The listing builds one solid part. Answer for the finished solid, in the listing's coordinates (mm). Face numbers are marked on the shaded views. Give positions to 0.01 mm unless a question says otherwise; leave off trailing zeros. Loops run counter-clockwise (first coordinate to the right, second up) from the corner with the lowest first, then second, coordinate; pieces in that order, holes last. Notation, with made-up numbers: (30, 6) -> (44, 6) arc R22 cw to (44, 40) -> close; hole circle Ø6 at (-32, 85.25). An arc over 180 degrees is marked (long way). One line per question, with ' | ' between items. Start each with the question number.
from build123d import *

# Parameters (mm, degrees)
SKETCH_1_W          = 206
SKETCH_1_H          = 215
EXTRUDE_1_DEPTH     = 15
SHELL_1_T           = -2
SKETCH_2_R          = 3
CUT_EXTRUDE_1_DEPTH = 15


with BuildPart() as part:
    # 草图1 → 凸台-拉伸1 (new body)
    with BuildSketch(Plane.XY):
        Rectangle(SKETCH_1_W, SKETCH_1_H)
    extrude(amount=EXTRUDE_1_DEPTH)

    # 抽壳1
    shell_1_openings = [part.faces().sort_by_distance(p)[0] for p in [
        (0, 0, 15),
    ]]
    offset(amount=SHELL_1_T, openings=shell_1_openings, kind=Kind.INTERSECTION)

    # 草图2 → 切除-拉伸1 (cut)
    with BuildSketch(Plane.XY.offset(2)):
        with Locations((-92, 0)):
            Circle(SKETCH_2_R)
        with Locations((0, 96.5)):
            Circle(SKETCH_2_R)
        with Locations((92, 0)):
            Circle(SKETCH_2_R)
        with Locations((0, -96.5)):
            Circle(SKETCH_2_R)
    extrude(amount=-CUT_EXTRUDE_1_DEPTH, mode=Mode.SUBTRACT)


solid = part.part
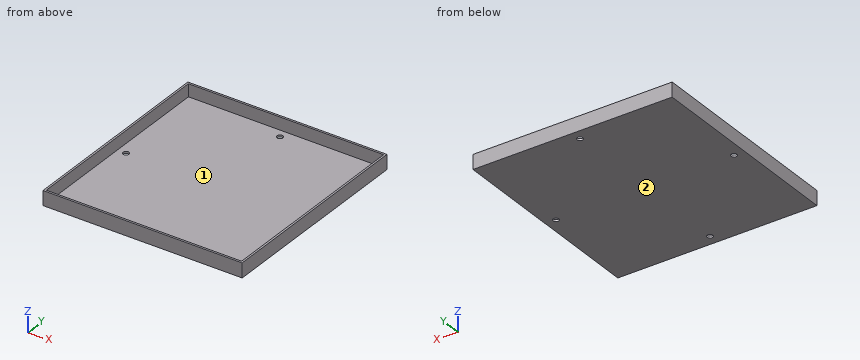
1. The part is cut by section C-C (x = -92). Write down the section's boundary in (y, z).
2. Straight lines are drawn through the part: L1, parallel to Y at x = 0, z = 1.3; L2, parallel to X at y = -70.5, z = 13.75; L3, parallel to Y at x = -49.5, z = 8. For each, find the intervals that lie inside material, in ascending order.
3. The part is cut by section D-D (z = 4.5). Write down the section's boundary in (x, y), plus the area to 3 significant figures.
4. This flat-tipped pin is pushed along its axis until it touches: pin 1 Ø2 at (x, y) = (48.5, -7.5) entering from +Z. Where does it stop, or does it pass through?
5. The part is cut by section B-B (y = 96.5). Write down the section's boundary in (x, z).
6. Determine the mould class of the marked faces 1 and 2 for opening direction X: released by +X, released by -X, zero draft, split by the parting line, or undercut.
7. The part is cut by section A-A (x = 0). Write down the section's boundary in (y, z).
Check sheet entries:
1) outline: (-107.5, 0) -> (-3, 0) -> (-3, 2) -> (-105.5, 2) -> (-105.5, 15) -> (-107.5, 15) -> close; (3, 0) -> (107.5, 0) -> (107.5, 15) -> (105.5, 15) -> (105.5, 2) -> (3, 2) -> close
2) L1: y = -107.5 to -99.5, -93.5 to 93.5, 99.5 to 107.5 | L2: x = -103 to -101, 101 to 103 | L3: y = -107.5 to -105.5, 105.5 to 107.5
3) outline: (-103, -107.5) -> (103, -107.5) -> (103, 107.5) -> (-103, 107.5) -> close; hole (-101, -105.5) -> (101, -105.5) -> (101, 105.5) -> (-101, 105.5) -> close | area: 1,670 mm^2
4) pin 1: stops at z = 2
5) outline: (-103, 0) -> (-3, 0) -> (-3, 2) -> (-101, 2) -> (-101, 15) -> (-103, 15) -> close; (3, 0) -> (103, 0) -> (103, 15) -> (101, 15) -> (101, 2) -> (3, 2) -> close
6) face 1: undercut | face 2: zero draft
7) outline: (-107.5, 0) -> (-99.5, 0) -> (-99.5, 2) -> (-105.5, 2) -> (-105.5, 15) -> (-107.5, 15) -> close; (-93.5, 0) -> (93.5, 0) -> (93.5, 2) -> (-93.5, 2) -> close; (99.5, 0) -> (107.5, 0) -> (107.5, 15) -> (105.5, 15) -> (105.5, 2) -> (99.5, 2) -> close
